Check sheet for the modelled part. Datum: model origin and axes. Units: mm. Face numbers are marked on the shaded views. A direction names the side the tool comes from. Round coordinates to 2 decimals unless told otherwise and drop trailing zeros. Order: outer loops, then holes, each group sorted by start corner. A loop starts at its lowest first (then second) coordinate and runs counter-clockwise, first axis right, second up.
(1) Depth check by flat-ended pin: pin 1 (4 mm diameter, centred on x = 2, y = 4.5, fed in from +Z); pin 2 (3 mm diameter, centred on x = 0, z = 34.12, fed in from +Y); pin 3 (1.6 mm diameter, centred on y = -2.5, z = 3, fed in from +X); pin 4 (3 mm diameter, centred on y = 6.5, z = 26.5, fed in from -X). Enter the tip coordinate at first touch or a pass-through.
(2) Thickness scan on probe 1 along X at (y, z) = (8.45, 34.12); probe 2 along Z at (x, y) = (17, 1); probe 3 along Y at (x, z) = (0.5, 29.5). Record the ranges inside material, lowest first.
(3) Sectioned sample at A-A, the plane z = 34.12. Enter the section's corners in (x, y).
(4) Sectioned sample at B-B, the plane x = 0. Enter the section's corners in (y, z).
(5) Sectioned sample at D-D, the plane z = 19. Enter the section's corners in (x, y), and give its area (3 significant figures).
(6) Tool access check on the marked faces 1, 2, 3 and 4. Record the directions out of +Z, -Z, +X, -X, +Y, -Y that give a thin tool (end or side, any length) a straight path to the whole face; none if there is none.
(7) Sectioned sample at C-C, the plane y = 4.5. Enter the section's corners in (x, z), and give its area (3 significant figures).
```python
from build123d import *

# Parameters (mm, degrees)
IZIM1_W                     = 44
IZIM1_H                     = 20
Y_KSEKLIK_EKSTR_ZYON1_DEPTH = 2
IZIM2_W                     = 42
IZIM2_H                     = 20
Y_KSEKLIK_EKSTR_ZYON2_DEPTH = 2
IZIM3_W                     = 10
IZIM3_H                     = 10
Y_KSEKLIK_EKSTR_ZYON3_DEPTH = 35
IZIM4_R                     = 2.52
KES_EKSTR_ZYON1_DEPTH       = 11
IZIM5_W                     = 10
IZIM5_H                     = 7.5
KES_EKSTR_ZYON2_DEPTH       = 9


with BuildPart() as part:
    # Çizim1 → Yükseklik-Ekstrüzyon1 (new body)
    with BuildSketch(Plane.XY):
        Rectangle(IZIM1_W, IZIM1_H)
    extrude(amount=Y_KSEKLIK_EKSTR_ZYON1_DEPTH)

    # Çizim2 → Yükseklik-Ekstrüzyon2 (add)
    with BuildSketch(Plane.XY.offset(2)):
        Rectangle(IZIM2_W, IZIM2_H)
    extrude(amount=Y_KSEKLIK_EKSTR_ZYON2_DEPTH)

    # Çizim3 → Yükseklik-Ekstrüzyon3 (add)
    with BuildSketch(Plane.XY.offset(4)):
        with Locations((0, 5)):
            Rectangle(IZIM3_W, IZIM3_H)
    extrude(amount=Y_KSEKLIK_EKSTR_ZYON3_DEPTH)

    # Çizim4 → Kes-Ekstrüzyon1 (cut)
    with BuildSketch(Plane(origin=(0, 10, 0), x_dir=(1, 0, 0), z_dir=(0, 1, 0))):
        with Locations(Location((0, -34.12, 0), (0, 0, 270))):
            Circle(IZIM4_R)
    extrude(amount=-KES_EKSTR_ZYON1_DEPTH, mode=Mode.SUBTRACT)

    # Çizim5 → Kes-Ekstrüzyon2 (cut)
    with BuildSketch(Plane.XY.offset(39)):
        with Locations((0, 3.75)):
            Rectangle(IZIM5_W, IZIM5_H)
    extrude(amount=-KES_EKSTR_ZYON2_DEPTH, mode=Mode.SUBTRACT)


solid = part.part
```
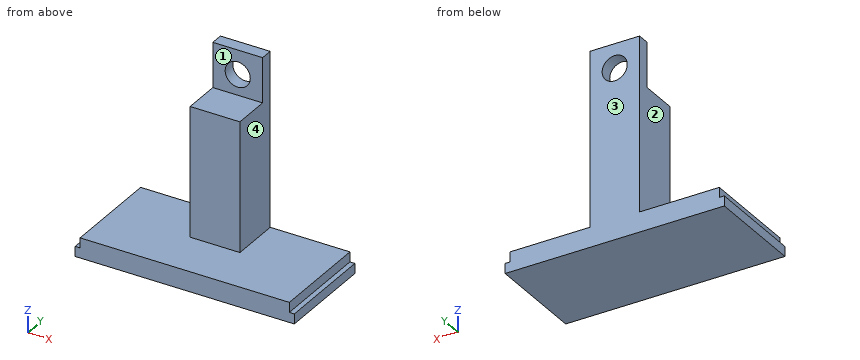
Derived:
1. pin 1: stops at z = 30
1. pin 2: passes through
1. pin 3: stops at x = 21
1. pin 4: stops at x = -5
2. probe 1: x = -5 to -2.52, 2.52 to 5
2. probe 2: z = 0 to 4
2. probe 3: y = 0 to 10
3. outline: (-5, 7.5) - (-2.52, 7.5) - (-2.52, 10) - (-5, 10) - close; (2.52, 7.5) - (5, 7.5) - (5, 10) - (2.52, 10) - close
4. outline: (-10, 0) - (10, 0) - (10, 31.6) - (7.5, 31.6) - (7.5, 30) - (0, 30) - (0, 4) - (-10, 4) - close; (7.5, 36.64) - (10, 36.64) - (10, 39) - (7.5, 39) - close
5. outline: (-5, 0) - (5, 0) - (5, 10) - (-5, 10) - close
5. area: 100 mm2
6. face 1: +Z, +X, -X, -Y
6. face 2: +Z, -X, +Y, -Y
6. face 3: +Z, -Z, +X, -X, +Y
6. face 4: +Z, +X, +Y, -Y
7. outline: (-22, 0) - (22, 0) - (22, 2) - (21, 2) - (21, 4) - (5, 4) - (5, 30) - (-5, 30) - (-5, 4) - (-21, 4) - (-21, 2) - (-22, 2) - close
7. area: 432 mm2
